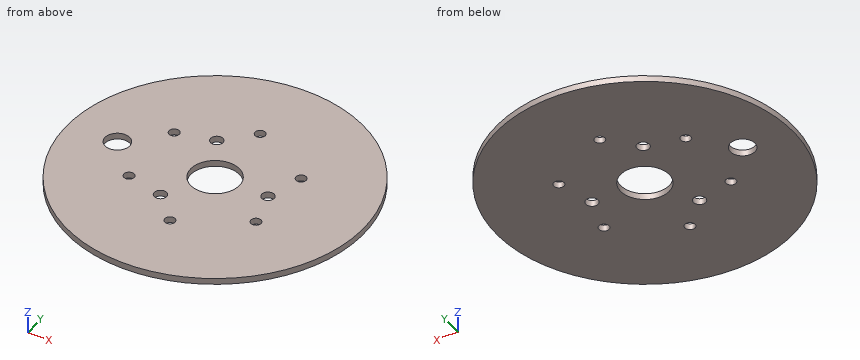
from build123d import *

# Parameters (mm, degrees)
SKETCH1_R           = 76.2
BOSS_EXTRUDE1_DEPTH = 3.175
CIRPATTERN1_COUNT   = 3
CIRPATTERN2_COUNT   = 6
SKETCH7_R           = 12.5
CUT_EXTRUDE2_DEPTH  = 4.175
SKETCH8_R           = 6.35
CUT_EXTRUDE3_DEPTH  = 4.175


with BuildPart() as part:
    # Sketch1 → Boss-Extrude1 (new body)
    with BuildSketch(Plane.XY):
        Circle(SKETCH1_R)
    extrude(amount=BOSS_EXTRUDE1_DEPTH)

    # Sketch4 → M5 Clearance Hole2 (revolve, cut)
    with BuildSketch(Plane(origin=(0, 38.1, 3.175), x_dir=(0, -1, 0), z_dir=(1, 0, 0))):
        Polygon((0, 0), (0, 14.03828064), (2.65, 12.446), (2.65, 0), align=None)
    m5_clearance_hole2 = revolve(axis=Axis((0, 38.1, 9.525), (0, 0, -1)), mode=Mode.SUBTRACT)

    # Sketch5 → M6 Clearance Hole1 (revolve, cut)
    with BuildSketch(Plane(origin=(-13.75, 23.815698604, 3.175), x_dir=(0, -1, 0), z_dir=(1, 0, 0))):
        Polygon((0, 0), (0, 14.368753981), (3.2, 12.446), (3.2, 0), align=None)
    m6_clearance_hole1 = revolve(axis=Axis((-13.75, 23.815698604, 9.525), (0, 0, -1)), mode=Mode.SUBTRACT)

    # CirPattern1: M6 Clearance Hole1 ×3 about axis
    cirpattern1_axis = Axis((0, 0, 0), (0, 0, 1))
    for i in range(1, CIRPATTERN1_COUNT):
        add(m6_clearance_hole1.rotate(cirpattern1_axis, i * 360 / CIRPATTERN1_COUNT), mode=Mode.SUBTRACT)

    # CirPattern2: M5 Clearance Hole2 ×6 about axis
    cirpattern2_axis = Axis((0, 0, 0), (0, 0, 1))
    for i in range(1, CIRPATTERN2_COUNT):
        add(m5_clearance_hole2.rotate(cirpattern2_axis, i * 360 / CIRPATTERN2_COUNT), mode=Mode.SUBTRACT)

    # Sketch7 → Cut-Extrude2 (cut, through all)
    with BuildSketch(Plane(origin=(0, 0, 0), x_dir=(-1, 0, 0), z_dir=(0, 0, -1))):
        Circle(SKETCH7_R)
    extrude(amount=-CUT_EXTRUDE2_DEPTH, mode=Mode.SUBTRACT)

    # Sketch8 → Cut-Extrude3 (cut, through all)
    with BuildSketch(Plane(origin=(0, 0, 0), x_dir=(-1, 0, 0), z_dir=(0, 0, -1))):
        with Locations((50.8, 0)):
            Circle(SKETCH8_R)
    extrude(amount=-CUT_EXTRUDE3_DEPTH, mode=Mode.SUBTRACT)


solid = part.part
Model file for the job. Use its own axes, mm. Coordinates: 2 decimals unless noted, no trailing zeros. Order: outer loops, then holes, each group sorted by start corner. A loop starts at its lowest first (then second) coordinate and runs counter-clockwise, first axis right, second up. Notation, with made-up numbers: (80.5, 40) -> (138.5, 40) arc R9 ccw to (138.5, 55) -> close; hole circle Ø6 at (44, -9). An arc over 180 degrees is marked (long way). Return JSON: item names as keys, results as strings. Group by question number.
Item 1: Flat gauge pins, fed straight in: P1, Ø6, axis at x = -13.75, y = -23.82, coming from the -Z side; P2, Ø7, axis at x = 33, y = -19.05, coming from the -Z side; P3, Ø1.5, axis at y = 11, z = 1, coming from the -X side; P4, Ø1, axis at y = -24.5, z = 2, coming from the +X side. Where does each tip first touch, or does it go through?
Item 2: Saw through at A-A on y = -38.1. Write the cut outline in (x, z) (3 decimals), then the cut area to 3 significant figures.
Item 3: Saw through at B-B on z = 0.75. State how many separate pieces and enclosed holes the cut face has, then the cut area to 3 significant figures.
Item 4: Saw through at D-D on y = 23.5. Write the cut outline in (x, z) (3 decimals).
Item 5: Wall check: line 1 along Y through (x, z) = (-11.5, 0.2); line 2 along Y through (x, z) = (0, 1.3); line 3 along X through (y, z) = (-19.05, 1.15). Give the ranges that are in metal, low to high. Write a range as [from, to].
Item 6: Saw through at C-C on x = 45. Write the cut outline in (y, z) (3 decimals).
Values found:
{
 "1": {"P1": "passes through", "P2": "stops at z = 0", "P3": "stops at x = -75.51", "P4": "stops at x = 72.32"},
 "2": {"outline": "(-65.991, 0) -> (-2.65, 0) -> (-2.65, 3.175) -> (-65.991, 3.175) -> close; (2.65, 0) -> (65.991, 0) -> (65.991, 3.175) -> (2.65, 3.175) -> close", "area": "402 mm2"},
 "3": {"separate pieces": "1", "enclosed holes": "11", "area": "17,400 mm2"},
 "4": {"outline": "(-72.486, 0) -> (-16.934, 0) -> (-16.934, 3.175) -> (-72.486, 3.175) -> close; (-10.566, 0) -> (72.486, 0) -> (72.486, 3.175) -> (-10.566, 3.175) -> close"},
 "5": {"line 1": "y = [-75.33, -26.09], [-21.54, -4.9], [4.9, 21.54], [26.09, 75.33]", "line 2": "y = [-76.2, -40.75], [-35.45, -12.5], [12.5, 35.45], [40.75, 76.2]", "line 3": "x = [-73.78, -35.65], [-30.35, 30.35], [35.65, 73.78]"},
 "6": {"outline": "(-61.493, 0) -> (61.493, 0) -> (61.493, 3.175) -> (-61.493, 3.175) -> close"}
}
